Input: part model. Units: mm. Frame: model coordinates. Face numbers are marked on the shaded views. A direction names the side the tool comes from. Round coordinates to 2 decimals unless told otherwise and drop trailing zeros. Write each loop counter-clockwise with the first axis right and the second up, starting at its lowest first coordinate (ties: lowest second). Pieces come first, ordered by that corner, then holes. Notation, with made-up numbers: M 32,-2 L 69,-2 A35 cw 69,32 Z; hole C 82.25,-10 d9. An arc over 180 degrees is marked long. Answer as CSV lines item,"result". Start each with the question number.
```python
from build123d import *

# Parameters (mm, degrees)
EXTRUDE_1_DEPTH          = 15
EXTRUDE_1_DEPTH_BACK     = 5
SKETCH_1_R               = 2.5
EXTRUDE_2_REACH          = 21.685
EXTRUDE_2_END_RADIUS     = 2.5
SKETCH_3_R               = 2.5
CUT_EXTRUDE_1_REACH      = 24.5
SKETCH_6_R               = 1
CUT_EXTRUDE_3_REACH      = 21.685
CUT_EXTRUDE_3_END_RADIUS = 1
SKETCH_7_R               = 1


with BuildPart() as part:
    # 草图1 → 凸台-拉伸1 (new, two sides: drawn at the far end of the back side and taken through both)
    with BuildSketch(Plane.XY.offset(-EXTRUDE_1_DEPTH_BACK)):
        Circle(SKETCH_1_R)
    extrude(amount=EXTRUDE_1_DEPTH + EXTRUDE_1_DEPTH_BACK)

    # 凸台-拉伸2: up to this cylinder (the profile starts outside it)
    extrude_2_end = Plane(origin=(0, 0, 5), z_dir=(0, 0, 1)) * Cylinder(EXTRUDE_2_END_RADIUS, 49.37, mode=Mode.PRIVATE)
    # 草图3 → 凸台-拉伸2 (add, up to the surface)
    with BuildSketch(Plane(origin=(0, 10, 0), x_dir=(1, 0, 0), z_dir=(0, 1, 0)), mode=Mode.PRIVATE) as extrude_2_sk1:
        with Locations(Location((0, -5, 0), (0, 0, 270))):
            Circle(SKETCH_3_R)
    extrude_2_tool1 = extrude(extrude_2_sk1.sketch, amount=-EXTRUDE_2_REACH, mode=Mode.PRIVATE) - extrude_2_end
    add(extrude_2_tool1.solids().sort_by_distance((0, 10, 5))[0])

    # 草图6 → 切除-拉伸1 (cut, up to next)
    with BuildSketch(Plane(origin=(0, 0, -5), x_dir=(-1, 0, 0), z_dir=(0, 0, -1)), mode=Mode.PRIVATE) as cut_extrude_1_sk1:
        Circle(SKETCH_6_R)
    cut_extrude_1_tool1 = extrude(cut_extrude_1_sk1.sketch, amount=-CUT_EXTRUDE_1_REACH, mode=Mode.PRIVATE) & part.part
    add(cut_extrude_1_tool1.solids().sort_by_distance((0, 0, -5))[0], mode=Mode.SUBTRACT)

    # 切除-拉伸3: up to this cylinder (the profile starts outside it)
    cut_extrude_3_end = Plane(origin=(0, 0, 5), z_dir=(0, 0, -1)) * Cylinder(CUT_EXTRUDE_3_END_RADIUS, 46.37, mode=Mode.PRIVATE)
    # 草图7 → 切除-拉伸3 (cut, up to the surface)
    with BuildSketch(Plane(origin=(0, 10, 0), x_dir=(1, 0, 0), z_dir=(0, 1, 0)), mode=Mode.PRIVATE) as cut_extrude_3_sk1:
        with Locations(Location((0, -5, 0), (0, 0, 270))):
            Circle(SKETCH_7_R)
    cut_extrude_3_tool1 = extrude(cut_extrude_3_sk1.sketch, amount=-CUT_EXTRUDE_3_REACH, mode=Mode.PRIVATE) - cut_extrude_3_end
    add(cut_extrude_3_tool1.solids().sort_by_distance((0, 10, 5))[0], mode=Mode.SUBTRACT)


solid = part.part
```
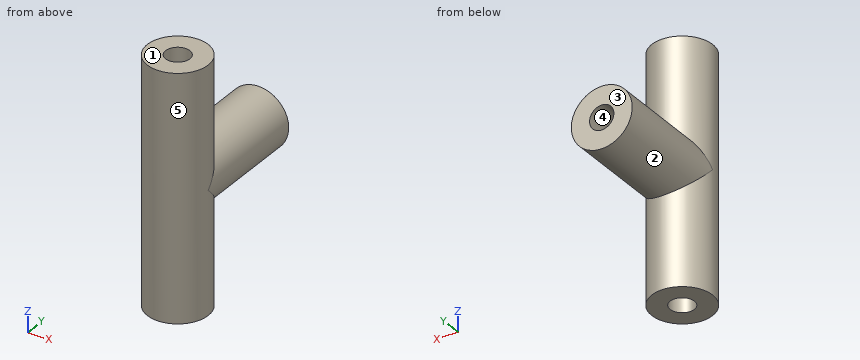
Item 1: Access query for the marked faces 1 and 2. Directions: +Z, -Z, +X, -X, +Y, -Y. A direction counts if a zero-diameter tool reaches every point of the face in a straight line with its end or side. Return the directions, or none.
Item 2: Cut plane C-C, the plane y = 7. Return loops of the section in (x, z), plus the area to 3 significant figures.
Item 3: Draft query along X for the marked faces 3, 4 and 5. Return one class per face: +X half, -X half, draft (parallel to the pull), parting line (faces both ways), or undercut.
Item 4: Cut plane A-A, the plane x = 0. Return loops of the section in (y, z), plus the area to 3 significant figures.
Item 5: Cut plane B-B, the plane z = 5. Return loops of the section in (x, y), plus the area to 3 significant figures.
Item 6: Cut plane D-D, the plane z = 0.5. Return loops of the section in (x, y).
Item 7: Line query: line 1 (X direction, y = 6.75, z = 5); line 2 (X direction, y = 0.5, z = 13); line 3 (Z direction, x = -0.15, y = 9). Output: solid intervals per line, ascending. Write a range as [from, to].
Item 8: Pin query (flat end, axial travel): pin 1 Ø3 at (y, z) = (3, 12) entering from -X; pin 2 Ø1 at (y, z) = (2.5, 10.5) entering from -X; pin 3 Ø3 at (x, z) = (1, 11.5) entering from +Y. Return the tip coordinate at first contact, or that it passes through.
Results list:
1,face 1,"+Z, +X, -X, +Y, -Y"
1,face 2,"+Y"
2,outline,"C 0,5 d5; hole C 0,5 d2"
2,area,"16.5 mm²"
3,face 3,"draft"
3,face 4,"undercut"
3,face 5,"parting line"
4,outline,"M -2.5,-5 L -1,-5 L -1,15 L -2.5,15 Z; M 1,-5 L 2.5,-5 L 2.5,2.5 L 10,2.5 L 10,4 L 1,4 Z; M 1,6 L 10,6 L 10,7.5 L 2.5,7.5 L 2.5,15 L 1,15 Z"
4,area,"79.5 mm²"
5,outline,"M -2.5,0 A2.5 ccw 2.5,0 L 2.5,10 L 1,10 L 1,0 A1 cw -1,0 L -1,10 L -2.5,10 Z"
5,area,"38.2 mm²"
6,outline,"C 0,0 d5; hole C 0,0 d2"
7,line 1,"[-2.5, -1], [1, 2.5]"
7,line 2,"[-2.45, -0.87], [0.87, 2.45]"
7,line 3,"[2.5, 4.01], [5.99, 7.5]"
8,pin 1,"x = -2"
8,pin 2,"x = -1.5"
8,pin 3,"y = 2.5"
